Geometry: final body of the model. Coordinates: model frame, mm. A direction names the side the tool comes from. Give positions to 0.01 mm unless a question says otherwise; leave off trailing zeros. Order: outer loops, then holes, each group sorted by start corner. A loop starts at its lowest first (then second) coordinate and runs counter-clockwise, first axis right, second up. Notation, with made-up numbers: (73, 65.25) - (107, 65.25) arc R13 ccw to (107, 90.25) - close; hole circle Ø9 at (77.25, -4). An arc over 180 degrees is marked (long way). One line per item, written item: value.
```python
from build123d import *

# Parameters (mm, degrees)
F1_DEPTH = 25.4
F2_DEPTH = 25.4
F3_DEPTH = 50.8


with BuildPart() as f1:
    # F0 (on Front) → F1 (new body)
    with BuildSketch(Plane.XZ):
        Polygon((-126.9120896435, -6.8535663185), (-160.2495896435, -6.8535663185), (-160.2495896435, -79.8785663185), (-7.8495896435, -79.8785663185), (-7.8495896435, -35.4285663185), (-126.9120896435, -35.4285663185), align=None)
    extrude(amount=F1_DEPTH)

    # F2 (add): a face of the model
    f2_faces = [f1.faces().sort_by_distance(p)[0] for p in [
        (-91.3890588215, -25.4, -53.1520252226),
    ]]
    extrude(f2_faces, amount=F2_DEPTH)

    # F3 (add): a face of the model
    f3_faces = [f1.faces().sort_by_distance(p)[0] for p in [
        (-91.3890588215, -50.8, -53.1520252226),
    ]]
    extrude(f3_faces, amount=F3_DEPTH)


solid = f1.part
```
1) Material intervals for line 1 along Z through (x, y) = (-33.5, -20.5); line 2 along X through (y, z) = (-93, -11), sorted ascending.
Answers below:
line 1: -79.88 to -35.43
line 2: -160.25 to -126.91
2) Section A-A, the plane y = -59. Return loops of the section in (x, z), then the cut area to 3 significant figures.
Answers below:
outline: (-160.25, -79.88) - (-7.85, -79.88) - (-7.85, -35.43) - (-126.91, -35.43) - (-126.91, -6.85) - (-160.25, -6.85) - close
area: 7,730 mm^2
3) First-contact query: pin 1 (3 mm diameter, centred on x = -42.5, y = -80.5, fed in from +Z); pin 2 (14.5 mm diameter, centred on y = -67, z = -20, fed in from +X). Flat tips, straight axial feed; report the tip coordinate or a pass-through.
Answers below:
pin 1: z = -35.43
pin 2: x = -126.91
4) Section B-B, the plane x = -75. Return loops of the section in (y, z).
Answers below:
outline: (-101.6, -79.88) - (0, -79.88) - (0, -35.43) - (-101.6, -35.43) - close
5) Set-up query: faces 1 (the face through (-160.25, -50, -43)), 2 (the face through (-126.912, -50, -21)). Return all of +Z, -Z, +X, -X, +Y, -Y with unobstructed straight access to the full face (end or side cutting, diameter ignored); none if empty.
Answers below:
face 1: +Z, -Z, -X, +Y, -Y
face 2: +Z, +X, +Y, -Y
6) Section C-C, the plane z = -32. Return loops of the section in (x, y), then the cut area to 3 significant figures.
Answers below:
outline: (-160.25, -101.6) - (-126.91, -101.6) - (-126.91, 0) - (-160.25, 0) - close
area: 3,390 mm^2
